from build123d import *

# Parameters (mm, degrees)
SKETCH1_R           = 2
BOSS_EXTRUDE2_DEPTH = 2.5


with BuildPart() as part:
    # Sketch1 → Boss-Extrude2 (new body, symmetric)
    with BuildSketch(Plane(origin=(0, 0, 0), x_dir=(1, 0, 0), z_dir=(0, 1, 0))):
        with BuildLine():
            Line((0, 0), (-6.495190528, -3.75))
            Line((-6.495190528, -3.75), (-6.745190528, -3.316987298))
            ThreePointArc((-6.745190528, -3.316987298), (-12.108900988, -8.267189567), (-4.845190528, -8.983012702))
            Line((-4.845190528, -8.983012702), (-5.095190528, -8.55))
            Line((-5.095190528, -8.55), (1.4, -4.8))
            ThreePointArc((1.4, -4.8), (4.191681084, -3.143760813), (5, 0))
            Line((5, 0), (5, 6))
            Line((5, 6), (0, 6))
            Line((0, 6), (0, 0))
        make_face()
        with Locations((-8.316447957, -6.99545846)):
            Circle(SKETCH1_R, mode=Mode.SUBTRACT)
    extrude(amount=BOSS_EXTRUDE2_DEPTH, both=True)


solid = part.part
Here's how the part is built. I have some questions about the finished solid (model axes, mm). A direction names the side the tool comes from. Coordinates: 2 decimals unless noted, no trailing zeros. Order: outer loops, then holes, each group sorted by start corner. A loop starts at its lowest first (then second) coordinate and runs counter-clockwise, first axis right, second up.
Item 1: If we section it at D-D on x = -3.25: List the corners of the cut face in (y, z) for me.
Result sheet:
outline: (-2.5, 1.88) - (2.5, 1.88) - (2.5, 7.48) - (-2.5, 7.48) - close
Item 2: If we section it at C-C on y = 0.3: List the corners of the cut face in (x, z) for me, plus the area to 3 significant figures.
Result sheet:
outline: (-6.75, 3.32) - (-6.5, 3.75) - (0, 0) - (0, -6) - (5, -6) - (5, 0) arc R4.25 ccw to (1.4, 4.8) - (-5.1, 8.55) - (-4.85, 8.98) arc R4 ccw (long way) to start; hole circle Ø4 at (-8.32, 7)
area: 116 mm2
Item 3: For faces 5 (the face through (-3.202, 0.035, 1.849)), 6 (the face through (-2, -2.5, 2)), which set-ups out of +Z, -Z, +X, -X, +Y, -Y let a thin tool reach every point of the face, with its end or its side?
Result sheet:
face 5: -Z, +Y, -Y
face 6: +Z, -Z, +X, -X, -Y
Item 4: I need wall thicknesses on line 1 (X direction, y = -0.75, z = -2.25); line 2 (Z direction, x = -7.75, y = -1.75); line 3 (X direction, y = -0.7, z = 8.25). Which ranges of each line are inside material? Lowest first, please.
Result sheet:
line 1: x = 0 to 5
line 2: z = 3.04 to 5.08, 8.91 to 10.96
line 3: x = -12.11 to -9.87, -6.76 to -4.58
Item 5: If we section it at B-B on x = -8.25: List the corners of the cut face in (y, z) for me, plus the area to 3 significant figures.
Result sheet:
outline: (-2.5, 3) - (2.5, 3) - (2.5, 5) - (-2.5, 5) - close; (-2.5, 8.99) - (2.5, 8.99) - (2.5, 10.99) - (-2.5, 10.99) - close
area: 20.0 mm2
Item 6: If we mould it in two halves opening along X, with no side actions, what happens to faces 1 (the face through (0, 0, -3)), 2 (the face through (3, 0, -6)), 3 (the face through (5, 0, -3)), 4 (the face through (-6.47, -0.04, 7.76))? For each: +X half, -X half, draft (parallel to the pull), parting line (faces both ways), or undercut.
Result sheet:
face 1: -X half
face 2: draft
face 3: +X half
face 4: undercut
Item 7: For P1, Ø2, axis at y = -1.5, z = -2.5, coming from the +X side; P2, Ø1, axis at y = -0.5, z = -4, coming from the -X side; P3, Ø2, axis at x = -1.5, y = 1, coming from the +Z side, each with a flat end and sliding along its axis, tell me the tip position at first contact or that it passes through.
Result sheet:
P1: stops at x = 5
P2: stops at x = 0
P3: stops at z = 7.05
Item 8: If we section it at A-A on z = 7.5: List the corners of the cut face in (x, y) for me, plus the area to 3 significant figures.
Result sheet:
outline: (-12.28, -2.5) - (-10.25, -2.5) - (-10.25, 2.5) - (-12.28, 2.5) - close; (-6.38, -2.5) - (-3.28, -2.5) - (-3.28, 2.5) - (-6.38, 2.5) - close
area: 25.7 mm2
